CAD build for the part. Positions are in the model's coordinates, mm. Coordinates: 2 decimals unless noted, no trailing zeros. Loops run counter-clockwise (first coordinate to the right, second up) from the corner with the lowest first, then second, coordinate; pieces in that order, holes last.
1) Wall check: line 1 along Z through (x, y) = (102, 4); line 2 along X through (y, z) = (5.5, 57); line 3 along Z through (x, y) = (-102.5, 6). Give the ranges that are in metal, low to high.
2) Saw through at C-C, the plane y = 1.75. Write the cut outline in (x, z), and give its area (3 significant figures).
3) Saw through at A-A, the plane z = 0. Write the cut outline in (x, y), and give its area (3 significant figures).
4) Saw through at B-B, the plane z = -57.5. Write the cut outline in (x, y).
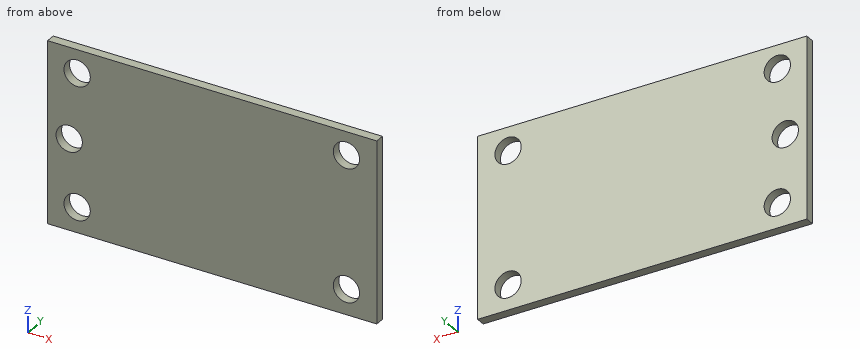
```python
from build123d import *

# Parameters (mm, degrees)
SKETCH4_W               = 250.263322682
SKETCH4_H               = 138.169331444
BOSS_EXTRUDE1_DEPTH     = 7
CUT_EXTRUDE1_DEPTH      = 60
CUT_EXTRUDE1_DEPTH_BACK = 144.107035844
SKETCH5_R               = 10
CUT_EXTRUDE6_DEPTH      = 68
CUT_EXTRUDE6_DEPTH_BACK = 76
SKETCH9_R               = 10


with BuildPart() as part:
    # Sketch4 → Boss-Extrude1 (new body)
    with BuildSketch(Plane(origin=(0, 0, 0), x_dir=(1, 0, 0), z_dir=(0, 1, 0))):
        Rectangle(SKETCH4_W, SKETCH4_H)
    extrude(amount=BOSS_EXTRUDE1_DEPTH)

    # Sketch5 → Cut-Extrude1 (cut, two sides: drawn at the far end of the back side and taken through both)
    with BuildSketch(Plane(origin=(0, 0, 0), x_dir=(1, 0, 0), z_dir=(0, 1, 0)).offset(-CUT_EXTRUDE1_DEPTH_BACK)):
        with Locations(Location((-102.685331177, 49.826038164, 0), (0, 0, 90))):
            Circle(SKETCH5_R)
        with Locations(Location((101.994027262, 49.826038164, 0), (0, 0, 90))):
            Circle(SKETCH5_R)
        with Locations(Location((101.994027262, -51.263637619, 0), (0, 0, 90))):
            Circle(SKETCH5_R)
        with Locations(Location((-102.685331177, -51.263637619, 0), (0, 0, 90))):
            Circle(SKETCH5_R)
    extrude(amount=CUT_EXTRUDE1_DEPTH + CUT_EXTRUDE1_DEPTH_BACK, mode=Mode.SUBTRACT)

    # Sketch9 → Cut-Extrude6 (cut, two sides: drawn at the far end of the back side and taken through both)
    with BuildSketch(Plane(origin=(0, 0, 0), x_dir=(1, 0, 0), z_dir=(0, 1, 0)).offset(-CUT_EXTRUDE6_DEPTH_BACK)):
        with Locations(Location((-108.72678805, 0, 0), (0, 0, 90))):
            Circle(SKETCH9_R)
    extrude(amount=CUT_EXTRUDE6_DEPTH + CUT_EXTRUDE6_DEPTH_BACK, mode=Mode.SUBTRACT)


solid = part.part
```
Data:
1. line 1: z = -69.08 to -59.83, -39.83 to 41.26, 61.26 to 69.08
1. line 2: x = -125.13 to -110.88, -94.49 to 93.8, 110.19 to 125.13
1. line 3: z = -69.08 to -59.82, -39.83 to -7.82, 7.82 to 41.27, 61.26 to 69.08
2. outline: (-125.13, -69.08) - (125.13, -69.08) - (125.13, 69.08) - (-125.13, 69.08) - close; hole circle Ø20 at (-108.73, 0); hole circle Ø20 at (-102.69, -49.83); hole circle Ø20 at (-102.69, 51.26); hole circle Ø20 at (101.99, -49.83); hole circle Ø20 at (101.99, 51.26)
2. area: 33,000 mm2
3. outline: (-125.13, 0) - (-118.73, 0) - (-118.73, 7) - (-125.13, 7) - close; (-98.73, 0) - (125.13, 0) - (125.13, 7) - (-98.73, 7) - close
3. area: 1,610 mm2
4. outline: (-125.13, 0) - (-109.1, 0) - (-109.1, 7) - (-125.13, 7) - close; (-96.27, 0) - (95.58, 0) - (95.58, 7) - (-96.27, 7) - close; (108.41, 0) - (125.13, 0) - (125.13, 7) - (108.41, 7) - close
